Could you check a few things on this drawing? It's one solid part, dimensions in mm from its lowest x, y, z. A direction names the side the tool comes from. Round coordinates to 2 decimals unless told otherwise and drop trailing zeros. Write each loop counter-clockwise with the first axis right and the second up, starting at its lowest first coordinate (ties: lowest second). Pieces come first, ordered by that corner, then holes. Notation, with made-up numbers: (-14, -19.75) - (-3, -19.75) arc R23 ccw to (-3, -10.75) - close; hole circle Ø5 at (8, -3). An arc over 180 degrees is marked (long way). One line per question, with ' | ' between items. Start each with the question number.
(1) Imagine slicing it at B-B (z = 9.5). Write out the boundary of the cut face in (x, y).
(2) Imagine slicing it at A-A (x = 60). Write out the boundary of the cut face in (y, z).
(3) For the marked faces 3 and 4, which set-ups out of +Z, -Z, +X, -X, +Y, -Y let a thin tool reach every point of the face, with its end or its side?
(4) Imagine slicing it at D-D (y = 19.5). Write out the boundary of the cut face in (x, z).
(5) Imagine slicing it at C-C (x = 7). Write out the boundary of the cut face in (y, z), plus the area to 3 significant figures.
(6) Thinking about a two-plate mould opening in X: for the marked faces 1 and 2, which applies, pulls with the +X half, pulls with the -X half, needs draft (parallel to the pull), parting line crosses it, or undercut?
(7) If I drill on L1, parallel to Y at x = 60, z = 5; L2, parallel to Y at x = 10, z = 17.75; L3, parallel to Z at x = 65.5, y = 2.25, over which ranges is the centre line in solid material (lowest first)?
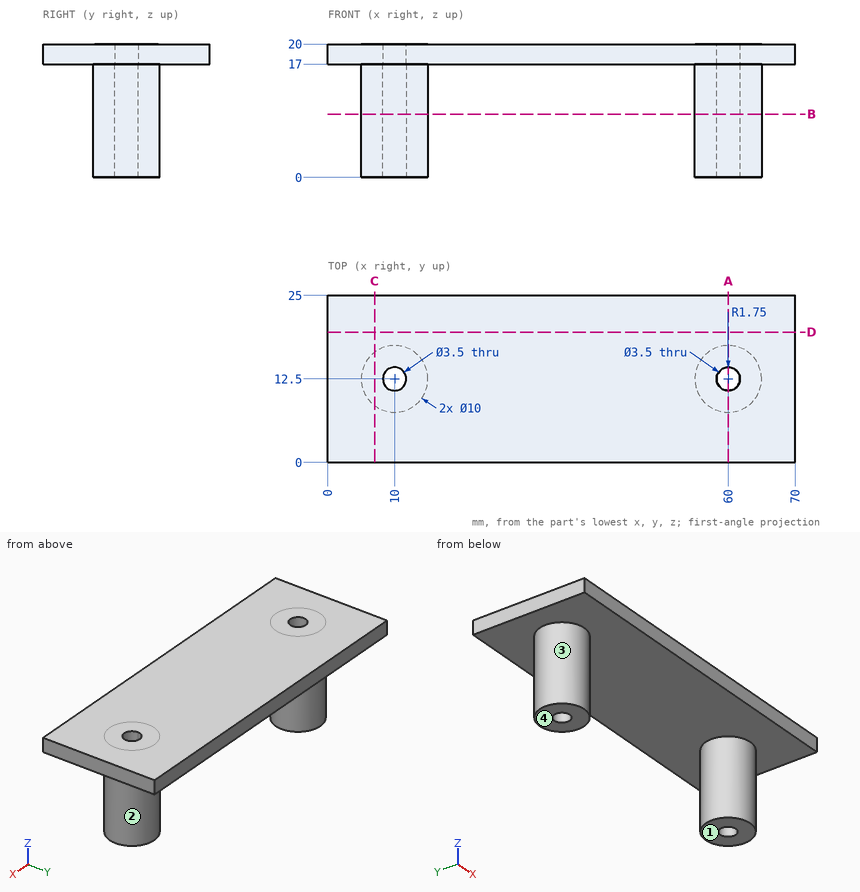
Check sheet entries:
1) outline: circle Ø10 at (10, 12.5); circle Ø10 at (60, 12.5); hole circle Ø3.5 at (10, 12.5); hole circle Ø3.5 at (60, 12.5)
2) outline: (0, 17) - (7.5, 17) - (7.5, 0) - (10.75, 0) - (10.75, 20) - (0, 20) - close; (14.25, 0) - (17.5, 0) - (17.5, 17) - (25, 17) - (25, 20) - (14.25, 20) - close
3) face 3: -Z | face 4: -Z, +X, -X, +Y, -Y
4) outline: (0, 17) - (70, 17) - (70, 20) - (0, 20) - close
5) outline: (0, 17) - (8.5, 17) - (8.5, 0) - (16.5, 0) - (16.5, 17) - (25, 17) - (25, 20) - (0, 20) - close | area: 211 mm^2
6) face 1: needs draft | face 2: undercut
7) L1: 7.5 to 10.75, 14.25 to 17.5 | L2: 0 to 10.75, 14.25 to 25 | L3: 17 to 20
